Can you work these out from the model? Positions are in its coordinate system, mm. Face numbers are marked on the shaded views. A direction names the side the tool comes from. Coordinates: 2 decimals unless noted, no trailing zeros. Order: outer loops, then holes, each group sorted by start corner. A loop starts at its lowest first (then second) coordinate and runs counter-clockwise, first axis right, second up. Notation, with made-up numbers: (64.5, -26) - (99.5, -26) arc R5 ccw to (99.5, -21) - close; hole circle Ø4 at (-4.5, -20). An arc over 180 degrees is marked (long way). Use a Markdown table: item, result. Add a question column.
(1) On a 3-axis mill with a long thin cutter (end or side, diameter ignored), from which of +Z, -Z, +X, -X, +Y, -Y can I reach the whole of each face in a straight line? I mean the marked faces 1 and 2. Say none if no direction works.
(2) We'd pull the mould along Z, two halves only. Please class the marked faces 3, 4 and 5: pulls with the +Z half, pulls with the -Z half, needs draft (parallel to the pull), parting line crosses it, or undercut.
(3) If I drill on L1, parallel to Z at x = 0, y = 1.25; L2, parallel to X at y = 0.85, z = 0; L3, parallel to Z at x = -5, y = 2.5, over which ranges is the centre line in solid material (lowest first)? Write a range as [from, to].
(4) For pin 1 Ø2 at (x, y) = (-1.5, 1.5) entering from +Z; pin 2 Ø1 at (x, y) = (-3.5, 2.5) entering from -Z; pin 3 Ø5 at (x, z) = (5.5, 3) entering from -Y; pin 4 Ø1.5 at (y, z) = (3, 4) entering from -X, each with a flat end and sliding along its axis, tell me the tip position at first contact or that it passes through.
(5) I want a section at B-B (x = 0). List the corners of the cut face in (y, z) for me, and give its area (3 significant figures).
(6) I want a section at A-A (z = 0). List the corners of the cut face in (x, y) for me, and give its area (3 significant figures).
Autodesk Inventor part; units mm, degrees
ref_plane "YZ Plane" through (0, 0, 0) normal (1, 0, 0) x (0, 1, 0)
ref_plane "XZ Plane" through (0, 0, 0) normal (0, 1, 0) x (-1, 0, 0)
ref_plane "XY Plane" through (0, 0, 0) normal (0, 0, 1) x (1, 0, 0)
sketch "Sketch1" plane through (0, 0, 0) normal (0, 1, 0) x (-1, 0, 0)
  circle A0 centre (0, 0) radius 4.1
  line L0 (6.3, 7.1) -> (-6.3, 7.1)
  line L1 (-6.3, 7.1) -> (-6.3, 5.1)
  line L2 (-6.3, 5.1) -> (6.3, 5.1)
  line L3 (6.3, 5.1) -> (6.3, 7.1)
  line L4 (6.3, 7.1) -> (-6.3, 5.1) construction
  line L5 (-6.3, 7.1) -> (6.3, 5.1) construction
  circle A1 centre (0, 0) radius 6.1
  line L6 (7.3, 8.1) -> (-7.3, 8.1)
  line L7 (-7.3, 8.1) -> (-7.3, 4.1)
  line L8 (-7.3, 4.1) -> (7.3, 4.1)
  line L9 (7.3, 4.1) -> (7.3, 8.1)
  point P0 (0, 6.1)
  point P1 (0, 6.1)
  point P2 (-4.5166, 4.1)
  point P3 (4.5166, 4.1)
  dimension "d0" = 8.2
  dimension "d1" = 12.6
  dimension "d2" = 2
  dimension "d3" = 1
  dimension "d4" = 1
  dimension "d5" = 2
extrude "Extrusion1" add sketch "Sketch1" along normal blind 4 contours L8 A1 | L8 A1 L2 | L8 L7 L6 L9 A1 L2 L3 L0 L1
fillet "Fillet1" radius 2 2 edges at (-4.5166, 2, 4.1) (4.5166, 2, 4.1)
fillet "Fillet2" radius 2 2 edges at (-7.3, 2, 4.1) (7.3, 2, 4.1)
fillet "Fillet3" radius 1 2 edges at (-7.3, 2, 8.1) (7.3, 2, 8.1)
sketch "Sketch2" plane through (0, 4, 0) normal (0, 1, 0) x (1, 0, 0)
  line L0 (6.3, -7.1) -> (-6.3, -7.1)
  line L1 (-6.3, -8.1) -> (6.3, -8.1)
  line L2 (-4.3, -7.1) -> (4.3, -7.1)
  line L3 (4.3, -7.1) -> (4.3, -8.1)
  line L4 (4.3, -8.1) -> (-4.3, -8.1)
  line L5 (-4.3, -8.1) -> (-4.3, -7.1)
  line L6 (-6.3, -7.1) -> (-6.3, -5.1)
  line L7 (6.3, -5.1) -> (6.3, -7.1)
  point P0 (0, 0)
  point P1 (4.3, -7.1)
  dimension "d11" = 2
  dimension "d12" = 2
extrude "Extrusion2" cut sketch "Sketch2" against normal through all
fillet "Fillet4" radius 0.5 4 edges at (-4.3, 2, 7.1) (-4.3, 2, 8.1) (4.3, 2, 7.1) (4.3, 2, 8.1)
fillet "Fillet5" radius 1 2 edges at (-6.3, 2, 7.1) (6.3, 2, 7.1)
fillet "Fillet6" radius 0.3 2 edges at (-6.3, 2, 5.1) (6.3, 2, 5.1)
properties part number "clip_rod" material "ABS Plastic"
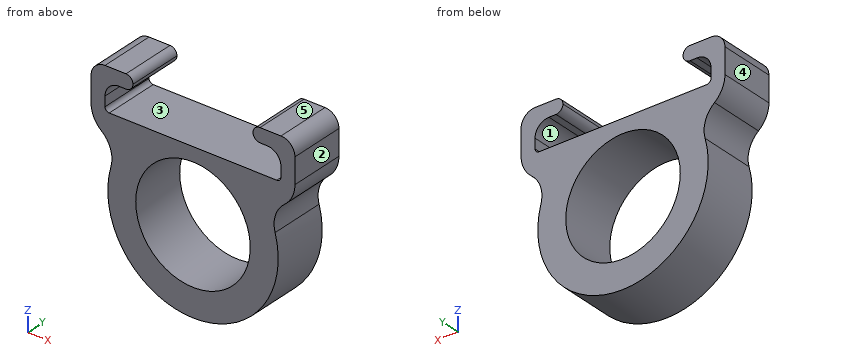
Answers follow:
| question | item | result |
|---|---|---|
| 1 | face 1 | +Y, -Y |
| 1 | face 2 | +Z, -Z, +X, +Y, -Y |
| 2 | face 3 | undercut |
| 2 | face 4 | needs draft |
| 2 | face 5 | pulls with the +Z half |
| 3 | L1 | z = [-6.1, -4.1], [4.1, 5.1] |
| 3 | L2 | x = [-6.1, -4.1], [4.1, 6.1] |
| 3 | L3 | z = [-3.49, 5.1], [7.1, 8.1] |
| 4 | pin 1 | stops at z = 5.1 |
| 4 | pin 2 | stops at z = -5.31 |
| 4 | pin 3 | stops at y = 0 |
| 4 | pin 4 | stops at x = -7.23 |
| 5 | outline | (0, -6.1) - (4, -6.1) - (4, -4.1) - (0, -4.1) - close; (0, 4.1) - (4, 4.1) - (4, 5.1) - (0, 5.1) - close |
| 5 | area | 12.0 mm² |
| 6 | outline | (-6.1, 0) - (-4.1, 0) - (-4.1, 4) - (-6.1, 4) - close; (4.1, 0) - (6.1, 0) - (6.1, 4) - (4.1, 4) - close |
| 6 | area | 16.0 mm² |
